The model under review builds one solid part; all positions refer to its coordinate system, in mm. A direction names the side the tool comes from. Round coordinates to 2 decimals unless told otherwise and drop trailing zeros. Loops run counter-clockwise (first coordinate to the right, second up) from the corner with the lowest first, then second, coordinate; pieces in that order, holes last. Notation, with made-up numbers: M 47,-32.75 L 84,-32.75 A15 cw 84,-20.75 Z; hole C -24,57 d11. An arc over 180 degrees is marked long. Return JSON: item names as keys, results as strings. Group by question number.
Q1. For faces 1 (the face through (-49.83, 1.48, 61.15)), 2 (the face through (-68, 1, -78)), list the 3-axis set-ups (+Z, -Z, +X, -X, +Y, -Y) from which the entire face can be reached by the end or side of a thin tool; tool diameter is ignored.
Q2. Consider section A-A (x = 0). State the section outline as (y, z) points, and give its area (3 significant figures).
Q3. To check wall thickness, follow line 1 along X through (y, z) = (1.55, 23.4); line 2 along X through (y, z) = (1.55, 72); line 3 along X through (y, z) = (0.65, 34.9). State the ranges of each line that lie inside material, in increasing order.
Q4. Consider section D-D (z = -46). State the section outline as (x, y) points.
Q5. Draft analysis for pull direction X (two halves, no side actions). For faces 3 (the face through (1, 0, -1)), 4 (the face through (-67, 1, 79)), 5 (the face through (0.1, 1.5, -35.1)), 6 (the face through (67, 1, -79)), state which applies: pulls with the +X half, pulls with the -X half, needs draft (parallel to the pull), parting line crosses it, or undercut.
Q6. Consider section B-B (y = 2.5). Count the separate pieces of the cut face and the enclosed holes in it, and give its area (3 significant figures).
Q7. Clearance check with flat-ended pins moving along their axes: pin 1 Ø3.5 at (x, z) = (-60, 72) entering from -Y; pin 2 Ø4 at (x, z) = (0, -32.5) entering from +Y. State where each tip first meets the part, or that it passes through.
Q8. Consider section C-C (x = -15.15). State the section outline as (y, z) points.
from build123d import *

# Parameters (mm, degrees)
SKETCH_1_R      = 1.6
SKETCH_1_R_2    = 11.1
SKETCH_1_R_3    = 1.5
SKETCH_1_R_4    = 11.25
SKETCH_1_R_5    = 2.6
EXTRUDE_1_DEPTH = 3


with BuildPart() as part:
    # 草图1 → 凸台-拉伸1 (new body)
    with BuildSketch(Plane(origin=(0, 0, 0), x_dir=(1, 0, 0), z_dir=(0, 1, 0))):
        with BuildLine():
            Line((64, -80), (-64, -80))
            ThreePointArc((-64, -80), (-67.535533906, -78.535533906), (-69, -75))
            Line((-69, -75), (-69, 75))
            ThreePointArc((-69, 75), (-67.535533906, 78.535533906), (-64, 80))
            Line((-64, 80), (64, 80))
            ThreePointArc((64, 80), (67.535533906, 78.535533906), (69, 75))
            Line((69, 75), (69, -75))
            ThreePointArc((69, -75), (67.535533906, -78.535533906), (64, -80))
        make_face()
        with Locations(Location((60, 76, 0), (0, 0, 270))):
            Circle(SKETCH_1_R, mode=Mode.SUBTRACT)
        with Locations(Location((-60, 76, 0), (0, 0, 90))):
            Circle(SKETCH_1_R, mode=Mode.SUBTRACT)
        with Locations(Location((0, -34.9, 0), (0, 0, 270))):
            Circle(SKETCH_1_R_2, mode=Mode.SUBTRACT)
        with Locations(Location((11.5, -46.4, 0), (0, 0, 270))):
            Circle(SKETCH_1_R_3, mode=Mode.SUBTRACT)
        with Locations(Location((11.5, -23.4, 0), (0, 0, 270))):
            Circle(SKETCH_1_R_3, mode=Mode.SUBTRACT)
        with Locations(Location((-11.5, -46.4, 0), (0, 0, 90))):
            Circle(SKETCH_1_R_3, mode=Mode.SUBTRACT)
        with Locations(Location((-11.5, -23.4, 0), (0, 0, 90))):
            Circle(SKETCH_1_R_3, mode=Mode.SUBTRACT)
        with Locations(Location((0, 50, 0), (0, 0, 270))):
            Circle(SKETCH_1_R_4, mode=Mode.SUBTRACT)
        with Locations(Location((60, -72, 0), (0, 0, 270))):
            Circle(SKETCH_1_R, mode=Mode.SUBTRACT)
        with Locations(Location((-60, -72, 0), (0, 0, 90))):
            Circle(SKETCH_1_R, mode=Mode.SUBTRACT)
        with Locations(Location((0, 32.5, 0), (0, 0, 270))):
            Circle(SKETCH_1_R_5, mode=Mode.SUBTRACT)
        with Locations(Location((15.15, 58.75, 0), (0, 0, 270))):
            Circle(SKETCH_1_R_5, mode=Mode.SUBTRACT)
        with Locations(Location((-15.15, 58.75, 0), (0, 0, 90))):
            Circle(SKETCH_1_R_5, mode=Mode.SUBTRACT)
        with BuildLine():
            Line((-42.1, -16.55), (-42.1, -53.25))
            ThreePointArc((-42.1, -53.25), (-50, -61.15), (-57.9, -53.25))
            Line((-57.9, -53.25), (-57.9, -16.55))
            ThreePointArc((-57.9, -16.55), (-50, -8.65), (-42.1, -16.55))
        make_face(mode=Mode.SUBTRACT)
    extrude(amount=EXTRUDE_1_DEPTH)


solid = part.part
Values:
{
 "1": {"face 1": "+Y, -Y", "face 2": "-Z, -X, +Y, -Y"},
 "2": {"outline": "M 0,-80 L 3,-80 L 3,-61.25 L 0,-61.25 Z; M 0,-38.75 L 3,-38.75 L 3,-35.1 L 0,-35.1 Z; M 0,-29.9 L 3,-29.9 L 3,23.8 L 0,23.8 Z; M 0,46 L 3,46 L 3,80 L 0,80 Z", "area": "330 mm2"},
 "3": {"line 1": "x = -69 to -57.9, -42.1 to -13, -10 to 10, 13 to 69", "line 2": "x = -69 to -61.6, -58.4 to 58.4, 61.6 to 69", "line 3": "x = -69 to -57.9, -42.1 to -11.1, 11.1 to 69"},
 "4": {"outline": "M -69,0 L -10.51,0 L -10.51,3 L -69,3 Z; M 10.51,0 L 69,0 L 69,3 L 10.51,3 Z"},
 "5": {"face 3": "needs draft", "face 4": "pulls with the -X half", "face 5": "undercut", "face 6": "pulls with the +X half"},
 "6": {"separate pieces": "1", "enclosed holes": "14", "area": "20,400 mm2"},
 "7": {"pin 1": "stops at y = 0", "pin 2": "passes through"},
 "8": {"outline": "M 0,-80 L 3,-80 L 3,-61.35 L 0,-61.35 Z; M 0,-56.15 L 3,-56.15 L 3,80 L 0,80 Z"}
}
